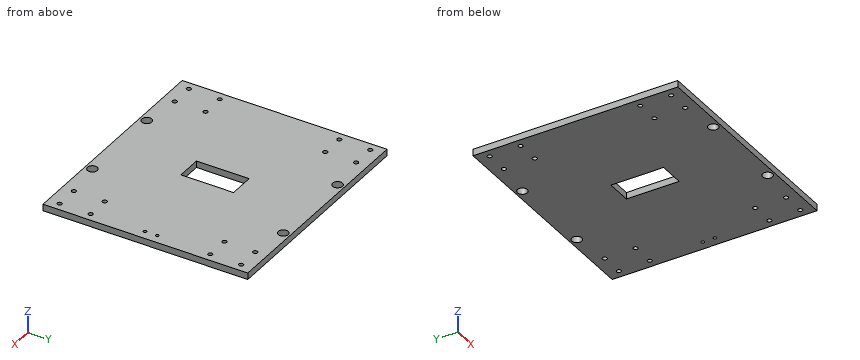
from build123d import *

# Parameters (mm, degrees)
F0_W     = 175.01715
F0_H     = 158.2801
F0_R     = 1.7272
F0_R_2   = 3.81
F0_R_3   = 1.25
F0_W_2   = 19.558
F0_H_2   = 40.64
F1_DEPTH = 5.08


with BuildPart() as f1:
    # F0 (on Top) → F1 (new body)
    with BuildSketch(Plane.XY):
        Rectangle(F0_W, F0_H)
        with Locations((-81.158575, -70.12305)):
            Circle(F0_R, mode=Mode.SUBTRACT)
        with Locations((-63.378575, -70.12305)):
            Circle(F0_R, mode=Mode.SUBTRACT)
        with Locations((-81.158575, -46.24705)):
            Circle(F0_R, mode=Mode.SUBTRACT)
        with Locations((-63.378575, -46.24705)):
            Circle(F0_R, mode=Mode.SUBTRACT)
        with Locations((-34.168575, -73.74255)):
            Circle(F0_R_2, mode=Mode.SUBTRACT)
        with Locations((34.168575, -73.74255)):
            Circle(F0_R_2, mode=Mode.SUBTRACT)
        with Locations((63.378575, -70.12305)):
            Circle(F0_R, mode=Mode.SUBTRACT)
        with Locations((81.158575, -70.12305)):
            Circle(F0_R, mode=Mode.SUBTRACT)
        with Locations((63.378575, -46.24705)):
            Circle(F0_R, mode=Mode.SUBTRACT)
        with Locations((81.158575, -46.24705)):
            Circle(F0_R, mode=Mode.SUBTRACT)
        with Locations((80.208564, -4.750003)):
            Circle(F0_R_3, mode=Mode.SUBTRACT)
        with Locations((-81.158575, 46.24705)):
            Circle(F0_R, mode=Mode.SUBTRACT)
        with Locations((-63.378575, 46.24705)):
            Circle(F0_R, mode=Mode.SUBTRACT)
        with Locations((-81.158575, 70.12305)):
            Circle(F0_R, mode=Mode.SUBTRACT)
        with Locations((-63.378575, 70.12305)):
            Circle(F0_R, mode=Mode.SUBTRACT)
        with Locations((-34.168575, 73.74255)):
            Circle(F0_R_2, mode=Mode.SUBTRACT)
        Rectangle(F0_W_2, F0_H_2, mode=Mode.SUBTRACT)
        with Locations((80.208564, 4.750003)):
            Circle(F0_R_3, mode=Mode.SUBTRACT)
        with Locations((34.168575, 73.74255)):
            Circle(F0_R_2, mode=Mode.SUBTRACT)
        with Locations((63.378575, 46.24705)):
            Circle(F0_R, mode=Mode.SUBTRACT)
        with Locations((81.158575, 46.24705)):
            Circle(F0_R, mode=Mode.SUBTRACT)
        with Locations((63.378575, 70.12305)):
            Circle(F0_R, mode=Mode.SUBTRACT)
        with Locations((81.158575, 70.12305)):
            Circle(F0_R, mode=Mode.SUBTRACT)
    extrude(amount=F1_DEPTH)


solid = f1.part
For this review, take the finished solid that the model builds, in its own axes (mm). Round coordinates to 2 decimals unless told otherwise and drop trailing zeros. Loops run counter-clockwise (first coordinate to the right, second up) from the corner with the lowest first, then second, coordinate; pieces in that order, holes last. Notation, with made-up numbers: (2.25, 69) - (21.25, 69) arc R30 ccw to (21.25, 100) - close; hole circle Ø9 at (-13, 17). An arc over 180 degrees is marked (long way). Use one line per item in the form item = value.
Item 1: Clearance check with flat-ended pins moving along their axes: P1, Ø4.5, axis at x = -81.16, y = 46.25, coming from the +Z side; P2, Ø3, axis at x = 63.38, y = -70.12, coming from the -Z side. State where each tip first meets the part, or that it passes through.
Answers:
P1 = 5.08
P2 = through
Item 2: Consider section A-A on y = -0.5. Write out the cut boundary in (x, z).
Answers:
outline = (-87.51, 0) - (-9.78, 0) - (-9.78, 5.08) - (-87.51, 5.08) - close; (9.78, 0) - (87.51, 0) - (87.51, 5.08) - (9.78, 5.08) - close
Item 3: Consider section B-B on x = 5. Write out the cut boundary in (y, z).
Answers:
outline = (-79.14, 0) - (-20.32, 0) - (-20.32, 5.08) - (-79.14, 5.08) - close; (20.32, 0) - (79.14, 0) - (79.14, 5.08) - (20.32, 5.08) - close
Item 4: For line 1 (X direction, y = -46.5, z = 3.8); line 2 (X direction, y = -5, z = 0.25), list the stretches that pass through material, from the lowest coordinate up.
Answers:
line_1 = -87.51 to -82.87, -79.45 to -65.09, -61.67 to 61.67, 65.09 to 79.45, 82.87 to 87.51
line_2 = -87.51 to -9.78, 9.78 to 78.98, 81.43 to 87.51
Item 5: Consider section C-C on z = 0.8. State how many separate pieces and enclosed holes the cut face has, then the cut area to 3 significant figures.
Answers:
separate_pieces = 1
enclosed_holes = 23
area = 26,600 mm^2
